from build123d import *

# Parameters (mm, degrees)
F1_DEPTH = 2.794
F2_R     = 10.311157
F3_DEPTH = 52.832
F4_R     = 7.62


with BuildPart() as f1:
    # F0 (on Front) → F1 (new body)
    with BuildSketch(Plane.XZ):
        with BuildLine():
            ThreePointArc((3.726169, 77.880541), (-73.645444, 75.509353), (-38.943787, 6.315538))
            ThreePointArc((-38.943787, 6.315538), (-40.482903, -37.881597), (3.726169, -36.735482))
            ThreePointArc((3.726169, -36.735482), (47.935241, -37.881597), (46.396125, 6.315538))
            ThreePointArc((46.396125, 6.315538), (81.097782, 75.509353), (3.726169, 77.880541))
        make_face()
    extrude(amount=-F1_DEPTH)

    # F2 (on Top) → F3 (join, symmetric)
    with BuildSketch(Plane.XY):
        with Locations((3.726171, 1.462447)):
            Circle(F2_R)
    extrude(amount=F3_DEPTH, both=True)

    # F4
    f4_edges = [f1.edges().sort_by_distance(p)[0] for p in [
        (3.726171, 11.773604, 52.832),
        (3.726171, -8.84871, 52.832),
        (-6.584986, 1.462447, -52.832),
    ]]
    fillet(f4_edges, radius=F4_R)


solid = f1.part
The listing builds one solid part. Answer for the finished solid, in the listing's coordinates (mm). Give positions to 0.01 mm unless a question says otherwise; leave off trailing zeros. Order: outer loops, then holes, each group sorted by start corner. A loop starts at its lowest first (then second) coordinate and runs counter-clockwise, first axis right, second up. Notation, with made-up numbers: (29, 15.25) - (50, 15.25) arc R14 cw to (50, 29.25) - close; hole circle Ø8 at (55.5, -5.5). An arc over 180 degrees is marked (long way). One line per item, written item: value. Start each with the question number.
1) Find the intervals of material crossed by L1, parallel to Y at x = 33.5, z = 37.5; L2, parallel to Z at x = 3.5, y = -0.25; L3, parallel to Z at x = -25.5, y = 2.75, in increasing order.
2) A cutting plane is placed at D-D on z = -24.5. Give the vertices of the cut face in (x, y).
3) A cutting plane is placed at A-A on z = 85. Give the vertices of the cut face in (x, y), then the cut area to 3 significant figures.
4) Given pin 1 Ø5 at (y, z) = (3.5, 40.5) entering from -X; pin 2 Ø3 at (y, z) = (-6, -13.5) entering from +X; pin 3 Ø1 at (x, y) = (3, -1) entering from +Z, each flat-ended and moving along its own axis, determine where each tip first touches the part or whether it passes through.
5) A cutting plane is placed at C-C on x = 74. Give the vertices of the cut face in (y, z).
6) A cutting plane is placed at B-B on z = 33. Give the vertices of the cut face in (x, y).
7) The mould has two halves that part along X. Classify faces 1 (the face through (-16, 2.794, 43)), 2 (the face through (-72.97, 1.38, 76.61)): released by +X, released by -X, zero draft, split by the parting line, or undercut.
Answer sheet:
1. L1: y = 0 to 2.79
1. L2: z = -52.83 to 52.83
1. L3: z = -46.15 to 97.08
2. outline: (-48.21, 0) - (-6.48, 0) arc R10.31 ccw to (13.93, 0) - (55.66, 0) - (55.66, 2.79) - (13.95, 2.79) arc R10.31 ccw to (-6.5, 2.79) - (-48.21, 2.79) - close
3. outline: (-66.13, 0) - (-2.28, 0) - (-2.28, 2.79) - (-66.13, 2.79) - close; (9.73, 0) - (73.58, 0) - (73.58, 2.79) - (9.73, 2.79) - close
3. area: 357 mm2
4. pin 1: stops at x = -79.21
4. pin 2: stops at x = 12.14
4. pin 3: stops at z = 52.83
5. outline: (0, 19.39) - (2.79, 19.39) - (2.79, 84.59) - (0, 84.59) - close
6. outline: (-76.01, 0) - (-6.48, 0) arc R10.31 ccw to (13.93, 0) - (83.47, 0) - (83.47, 2.79) - (13.95, 2.79) arc R10.31 ccw to (-6.5, 2.79) - (-76.01, 2.79) - close
7. face 1: zero draft
7. face 2: undercut
